Could you check a few things on this model? Use its own coordinates, in mm. A direction names the side the tool comes from. Coordinates: 2 decimals unless noted, no trailing zeros. Write each loop counter-clockwise with the first axis right and the second up, starting at its lowest first coordinate (ties: lowest second). Pieces come first, ordered by that corner, then holes. Notation, with made-up numbers: M 9.25,71.25 L 20.25,71.25 A23 ccw 20.25,80.25 Z; hole C 59,87.25 d4. An arc over 180 degrees is marked long. Answer as CSV lines item,"result". Start each with the question number.
Item 1: On a 3-axis mill with a long thin cutter (end or side, diameter ignored), from which of +Z, -Z, +X, -X, +Y, -Y can I reach the whole of each face in a straight line? I mean faces 1 (the flat face through (-5, -15, 1)), 2 (the flat face through (6.5, -6.5, 95)). Say none if no direction works.
Item 2: Suppose I cut it at D-D, the plane y = -10.5. Write out the boundary of the cut face in (x, z).
Item 3: I'm going to push flat-ended pins straight in: P1, Ø2, axis at x = -2, z = 80.5, coming from the +Y side; P2, Ø4, axis at x = 3.5, z = 55, coming from the -Y side; P3, Ø4, axis at y = -3.5, z = 46, coming from the +X side; P4, Ø4, axis at x = 1.5, y = -4.5, coming from the -Z side. Where does each tip first touch, or does it pass through?
Item 4: Suppose I cut it at B-B, the plane x = 3.5. Write out the boundary of the cut face in (y, z), and give its area (3 significant figures).
Item 5: Suppose I cut it at C-C, the plane z = 35.5. Write out the boundary of the cut face in (x, y), and give its area (3 significant figures).
Item 6: Suppose I cut it at A-A, the plane y = 5. Write out the boundary of the cut face in (x, z).
Item 7: If I drill on line 1 along Z through (x, y) = (-3.5, 10.5); line 2 along Z through (x, y) = (-19.5, -7); line 3 along X through (y, z) = (7, 35.5), over which ranges is the centre line in solid material (lowest first)? Write a range as [from, to].
```python
from build123d import *

# Parameters (mm, degrees)
F1_DEPTH = 3
F2_DEPTH = 95
F3_DEPTH = 115


with BuildPart() as f1:
    # F0 (on Top) → F1 (new body)
    with BuildSketch(Plane.XY):
        with BuildLine():
            ThreePointArc((0, -15), (-15, 0), (0, 15))
            Line((0, 15), (-10, 15))
            ThreePointArc((-10, 15), (-25, 0), (-10, -15))
            Line((-10, -15), (0, -15))
        make_face()
        with BuildLine():
            ThreePointArc((0, -15), (10.606602, -10.606602), (15, 0))
            ThreePointArc((15, 0), (10.606602, 10.606602), (0, 15))
            ThreePointArc((0, 15), (-15, 0), (0, -15))
        make_face()
        with BuildLine():
            ThreePointArc((-8.5, 0), (0, 8.5), (8.5, 0))
            ThreePointArc((8.5, 0), (0, -8.5), (-8.5, 0))
        make_face(mode=Mode.SUBTRACT)
        with BuildLine():
            ThreePointArc((-8.5, 0), (0, -8.5), (8.5, 0))
            ThreePointArc((8.5, 0), (0, 8.5), (-8.5, 0))
        make_face()
    extrude(amount=F1_DEPTH)

    # F0 (on Top) → F2 (join)
    with BuildSketch(Plane.XY):
        with BuildLine():
            ThreePointArc((0, -15), (10.606602, -10.606602), (15, 0))
            ThreePointArc((15, 0), (10.606602, 10.606602), (0, 15))
            ThreePointArc((0, 15), (-15, 0), (0, -15))
        make_face()
        with BuildLine():
            ThreePointArc((-8.5, 0), (0, 8.5), (8.5, 0))
            ThreePointArc((8.5, 0), (0, -8.5), (-8.5, 0))
        make_face(mode=Mode.SUBTRACT)
        with BuildLine():
            ThreePointArc((-8.5, 0), (0, -8.5), (8.5, 0))
            ThreePointArc((8.5, 0), (0, 8.5), (-8.5, 0))
        make_face()
    extrude(amount=F2_DEPTH)

    # F0 (on Top) → F3 (join)
    with BuildSketch(Plane.XY):
        with BuildLine():
            ThreePointArc((-8.5, 0), (0, -8.5), (8.5, 0))
            ThreePointArc((8.5, 0), (0, 8.5), (-8.5, 0))
        make_face()
    extrude(amount=F3_DEPTH)


solid = f1.part
```
Ans:
1,face 1,"+Z, -Z, +X, -X, -Y"
1,face 2,"+Z"
2,outline,"M -20.71,0 L 10.71,0 L 10.71,95 L -10.71,95 L -10.71,3 L -20.71,3 Z"
3,P1,"stops at y = 14.97"
3,P2,"stops at y = -14.92"
3,P3,"stops at x = 14.92"
3,P4,"stops at z = 0"
4,outline,"M -14.59,0 L 14.59,0 L 14.59,95 L 7.75,95 L 7.75,115 L -7.75,115 L -7.75,95 L -14.59,95 Z"
4,area,"3,080 mm^2"
5,outline,"M 0,-15 A15 ccw 15,0 A15 ccw long Z"
5,area,"707 mm^2"
6,outline,"M -24.14,0 L 14.14,0 L 14.14,95 L 6.87,95 L 6.87,115 L -6.87,115 L -6.87,95 L -14.14,95 L -14.14,3 L -24.14,3 Z"
7,line 1,"z = [0, 95]"
7,line 2,"z = [0, 3]"
7,line 3,"x = [-13.27, 13.27]"
